For this review, take the finished solid that the model builds, in its own axes (mm). Give positions to 0.01 mm unless a question says otherwise; leave off trailing zeros. Write each question's results on one line, items separated by ' | '. Start each with the question number.
```python
from build123d import *

# Parameters (mm, degrees)
SKETCH1_R           = 2.1463
BOSS_EXTRUDE1_DEPTH = 304.8


with BuildPart() as part:
    # Sketch1 → Boss-Extrude1 (new, symmetric)
    with BuildSketch(Plane.XY):
        with BuildLine():
            Line((-19.9898, 7.9883), (-19.9898, 3.2893))
            ThreePointArc((-19.9898, 3.2893), (-19.75917588, 2.73252412), (-19.2024, 2.5019))
            Line((-19.2024, 2.5019), (-18.4912, 2.5019))
            ThreePointArc((-18.4912, 2.5019), (-18.275673853, 2.591173853), (-18.1864, 2.8067))
            Line((-18.1864, 2.8067), (-18.1864, 4.9149))
            ThreePointArc((-18.1864, 4.9149), (-17.668965253, 5.689295824), (-16.755503096, 5.507596904))
            Line((-16.755503096, 5.507596904), (-14.500665747, 3.252759555))
            ThreePointArc((-14.500665747, 3.252759555), (-13.850954457, 2.280397894), (-13.622806192, 1.133419111))
            Line((-13.622806192, 1.133419111), (-13.622806192, -1.133419111))
            ThreePointArc((-13.622806192, -1.133419111), (-13.850954457, -2.280397894), (-14.500665747, -3.252759555))
            Line((-14.500665747, -3.252759555), (-16.755503096, -5.507596904))
            ThreePointArc((-16.755503096, -5.507596904), (-17.668965253, -5.689295824), (-18.1864, -4.9149))
            Line((-18.1864, -4.9149), (-18.1864, -2.8067))
            ThreePointArc((-18.1864, -2.8067), (-18.275673853, -2.591173853), (-18.4912, -2.5019))
            Line((-18.4912, -2.5019), (-19.2024, -2.5019))
            ThreePointArc((-19.2024, -2.5019), (-19.75917588, -2.73252412), (-19.9898, -3.2893))
            Line((-19.9898, -3.2893), (-19.9898, -7.9883))
            ThreePointArc((-19.9898, -7.9883), (-19.402080467, -9.407180467), (-17.9832, -9.9949))
            Line((-17.9832, -9.9949), (-13.2842, -9.9949))
            ThreePointArc((-13.2842, -9.9949), (-12.72742412, -9.76427588), (-12.4968, -9.2075))
            Line((-12.4968, -9.2075), (-12.4968, -8.4963))
            ThreePointArc((-12.4968, -8.4963), (-12.586073853, -8.280773853), (-12.8016, -8.1915))
            Line((-12.8016, -8.1915), (-14.9098, -8.1915))
            ThreePointArc((-14.9098, -8.1915), (-15.684195824, -7.674065253), (-15.502496904, -6.760603096))
            Line((-15.502496904, -6.760603096), (-13.247659555, -4.505765747))
            ThreePointArc((-13.247659555, -4.505765747), (-12.275297894, -3.856054457), (-11.128319111, -3.627906192))
            Line((-11.128319111, -3.627906192), (-8.861480889, -3.627906192))
            ThreePointArc((-8.861480889, -3.627906192), (-7.714502106, -3.856054457), (-6.742140445, -4.505765747))
            Line((-6.742140445, -4.505765747), (-4.487303096, -6.760603096))
            ThreePointArc((-4.487303096, -6.760603096), (-4.305604176, -7.674065253), (-5.08, -8.1915))
            Line((-5.08, -8.1915), (-7.1882, -8.1915))
            ThreePointArc((-7.1882, -8.1915), (-7.403726147, -8.280773853), (-7.493, -8.4963))
            Line((-7.493, -8.4963), (-7.493, -9.2075))
            ThreePointArc((-7.493, -9.2075), (-7.26237588, -9.76427588), (-6.7056, -9.9949))
            Line((-6.7056, -9.9949), (0, -9.9949))
            Line((0, -9.9949), (6.7056, -9.9949))
            ThreePointArc((6.7056, -9.9949), (7.26237588, -9.76427588), (7.493, -9.2075))
            Line((7.493, -9.2075), (7.493, -8.4963))
            ThreePointArc((7.493, -8.4963), (7.403726147, -8.280773853), (7.1882, -8.1915))
            Line((7.1882, -8.1915), (5.08, -8.1915))
            ThreePointArc((5.08, -8.1915), (4.305604176, -7.674065253), (4.487303096, -6.760603096))
            Line((4.487303096, -6.760603096), (6.742140445, -4.505765747))
            ThreePointArc((6.742140445, -4.505765747), (7.714502106, -3.856054457), (8.861480889, -3.627906192))
            Line((8.861480889, -3.627906192), (11.128319111, -3.627906192))
            ThreePointArc((11.128319111, -3.627906192), (12.275297894, -3.856054457), (13.247659555, -4.505765747))
            Line((13.247659555, -4.505765747), (15.502496904, -6.760603096))
            ThreePointArc((15.502496904, -6.760603096), (15.684195824, -7.674065253), (14.9098, -8.1915))
            Line((14.9098, -8.1915), (12.8016, -8.1915))
            ThreePointArc((12.8016, -8.1915), (12.586073853, -8.280773853), (12.4968, -8.4963))
            Line((12.4968, -8.4963), (12.4968, -9.2075))
            ThreePointArc((12.4968, -9.2075), (12.72742412, -9.76427588), (13.2842, -9.9949))
            Line((13.2842, -9.9949), (17.9832, -9.9949))
            ThreePointArc((17.9832, -9.9949), (19.402080467, -9.407180467), (19.9898, -7.9883))
            Line((19.9898, -7.9883), (19.9898, -3.2893))
            ThreePointArc((19.9898, -3.2893), (19.75917588, -2.73252412), (19.2024, -2.5019))
            Line((19.2024, -2.5019), (18.4912, -2.5019))
            ThreePointArc((18.4912, -2.5019), (18.275673853, -2.591173853), (18.1864, -2.8067))
            Line((18.1864, -2.8067), (18.1864, -4.9149))
            ThreePointArc((18.1864, -4.9149), (17.668965253, -5.689295824), (16.755503096, -5.507596904))
            Line((16.755503096, -5.507596904), (14.500665747, -3.252759555))
            ThreePointArc((14.500665747, -3.252759555), (13.850954457, -2.280397894), (13.622806192, -1.133419111))
            Line((13.622806192, -1.133419111), (13.622806192, 1.133419111))
            ThreePointArc((13.622806192, 1.133419111), (13.850954457, 2.280397894), (14.500665747, 3.252759555))
            Line((14.500665747, 3.252759555), (16.755503096, 5.507596904))
            ThreePointArc((16.755503096, 5.507596904), (17.668965253, 5.689295824), (18.1864, 4.9149))
            Line((18.1864, 4.9149), (18.1864, 2.8067))
            ThreePointArc((18.1864, 2.8067), (18.275673853, 2.591173853), (18.4912, 2.5019))
            Line((18.4912, 2.5019), (19.2024, 2.5019))
            ThreePointArc((19.2024, 2.5019), (19.75917588, 2.73252412), (19.9898, 3.2893))
            Line((19.9898, 3.2893), (19.9898, 7.9883))
            ThreePointArc((19.9898, 7.9883), (19.402080467, 9.407180467), (17.9832, 9.9949))
            Line((17.9832, 9.9949), (13.2842, 9.9949))
            ThreePointArc((13.2842, 9.9949), (12.72742412, 9.76427588), (12.4968, 9.2075))
            Line((12.4968, 9.2075), (12.4968, 8.4963))
            ThreePointArc((12.4968, 8.4963), (12.586073853, 8.280773853), (12.8016, 8.1915))
            Line((12.8016, 8.1915), (14.9098, 8.1915))
            ThreePointArc((14.9098, 8.1915), (15.684195824, 7.674065253), (15.502496904, 6.760603096))
            Line((15.502496904, 6.760603096), (13.247659555, 4.505765747))
            ThreePointArc((13.247659555, 4.505765747), (12.275297894, 3.856054457), (11.128319111, 3.627906192))
            Line((11.128319111, 3.627906192), (8.861480889, 3.627906192))
            ThreePointArc((8.861480889, 3.627906192), (7.714502106, 3.856054457), (6.742140445, 4.505765747))
            Line((6.742140445, 4.505765747), (4.487303096, 6.760603096))
            ThreePointArc((4.487303096, 6.760603096), (4.305604176, 7.674065253), (5.08, 8.1915))
            Line((5.08, 8.1915), (7.1882, 8.1915))
            ThreePointArc((7.1882, 8.1915), (7.403726147, 8.280773853), (7.493, 8.4963))
            Line((7.493, 8.4963), (7.493, 9.2075))
            ThreePointArc((7.493, 9.2075), (7.26237588, 9.76427588), (6.7056, 9.9949))
            Line((6.7056, 9.9949), (0, 9.9949))
            Line((0, 9.9949), (-6.7056, 9.9949))
            ThreePointArc((-6.7056, 9.9949), (-7.26237588, 9.76427588), (-7.493, 9.2075))
            Line((-7.493, 9.2075), (-7.493, 8.4963))
            ThreePointArc((-7.493, 8.4963), (-7.403726147, 8.280773853), (-7.1882, 8.1915))
            Line((-7.1882, 8.1915), (-5.08, 8.1915))
            ThreePointArc((-5.08, 8.1915), (-4.305604176, 7.674065253), (-4.487303096, 6.760603096))
            Line((-4.487303096, 6.760603096), (-6.742140445, 4.505765747))
            ThreePointArc((-6.742140445, 4.505765747), (-7.714502106, 3.856054457), (-8.861480889, 3.627906192))
            Line((-8.861480889, 3.627906192), (-11.128319111, 3.627906192))
            ThreePointArc((-11.128319111, 3.627906192), (-12.275297894, 3.856054457), (-13.247659555, 4.505765747))
            Line((-13.247659555, 4.505765747), (-15.502496904, 6.760603096))
            ThreePointArc((-15.502496904, 6.760603096), (-15.684195824, 7.674065253), (-14.9098, 8.1915))
            Line((-14.9098, 8.1915), (-12.8016, 8.1915))
            ThreePointArc((-12.8016, 8.1915), (-12.586073853, 8.280773853), (-12.4968, 8.4963))
            Line((-12.4968, 8.4963), (-12.4968, 9.2075))
            ThreePointArc((-12.4968, 9.2075), (-12.72742412, 9.76427588), (-13.2842, 9.9949))
            Line((-13.2842, 9.9949), (-17.9832, 9.9949))
            ThreePointArc((-17.9832, 9.9949), (-19.402080467, 9.407180467), (-19.9898, 7.9883))
        make_face()
        with Locations((-9.9949, 0)):
            Circle(SKETCH1_R, mode=Mode.SUBTRACT)
        with Locations(Location((9.9949, 0, 0), (0, 0, 180))):
            Circle(SKETCH1_R, mode=Mode.SUBTRACT)
        with BuildLine():
            Line((-6.366993808, 1.133419111), (-6.366993808, -1.133419111))
            ThreePointArc((-6.366993808, -1.133419111), (-6.138845543, -2.280397894), (-5.489134253, -3.252759555))
            Line((-5.489134253, -3.252759555), (-0.939581002, -7.802312806))
            ThreePointArc((-0.939581002, -7.802312806), (0, -8.1915), (0.939581002, -7.802312806))
            Line((0.939581002, -7.802312806), (5.489134253, -3.252759555))
            ThreePointArc((5.489134253, -3.252759555), (6.138845543, -2.280397894), (6.366993808, -1.133419111))
            Line((6.366993808, -1.133419111), (6.366993808, 1.133419111))
            ThreePointArc((6.366993808, 1.133419111), (6.138845543, 2.280397894), (5.489134253, 3.252759555))
            Line((5.489134253, 3.252759555), (0.939581002, 7.802312806))
            ThreePointArc((0.939581002, 7.802312806), (0, 8.1915), (-0.939581002, 7.802312806))
            Line((-0.939581002, 7.802312806), (-5.489134253, 3.252759555))
            ThreePointArc((-5.489134253, 3.252759555), (-6.138845543, 2.280397894), (-6.366993808, 1.133419111))
        make_face(mode=Mode.SUBTRACT)
    extrude(amount=BOSS_EXTRUDE1_DEPTH, both=True)


solid = part.part
```
1. For pin 1 Ø0.6 at (y, z) = (8.5, 59) entering from -X; pin 2 Ø2 at (y, z) = (0, 103.5) entering from -X; pin 3 Ø0.6 at (y, z) = (9, 17.5) entering from +X, all flat-tipped, find the tip position at first contact; note any pin that passes through.
2. We need section A-A (z = 23). Count the separate pieces of the cut face and the enclosed holes in it, plus the area to 4 significant figures.
3. Wall thickness on L1, parallel to Y at x = 13, z = 253; L2, parallel to X at y = -0.25, z = -111.5; L3, parallel to X at y = 6.25, z = 25: over which ranges is each line inside the solid? List them lowest first.
Response:
1) pin 1: stops at x = -19.98 | pin 2: stops at x = -13.62 | pin 3: stops at x = 19.86
2) separate pieces: 1 | enclosed holes: 3 | area: 328.5 mm2
3) L1: y = -9.94 to -8.19, -4.28 to 4.28, 8.19 to 9.94 | L2: x = -13.62 to -12.13, -7.86 to -6.37, 6.37 to 7.86, 12.13 to 13.62 | L3: x = -19.99 to -14.99, -5 to -2.49, 2.49 to 5, 14.99 to 19.99
